from build123d import *

# Parameters (mm, degrees)
SKETCH1_R           = 10
BOSS_EXTRUDE1_DEPTH = 10


with BuildPart() as part:
    # Sketch1 → Boss-Extrude1 (new body)
    with BuildSketch(Plane.XY):
        with BuildLine():
            Line((-89.519341996, 20), (310.480658004, 20))
            ThreePointArc((310.480658004, 20), (330.480658004, 0), (310.480658004, -20))
            Line((310.480658004, -20), (-89.519341996, -20))
            ThreePointArc((-89.519341996, -20), (-109.519341996, 0), (-89.519341996, 20))
        make_face()
        with Locations((-89.519341996, 0)):
            Circle(SKETCH1_R, mode=Mode.SUBTRACT)
        with Locations((310.480658004, 0)):
            Circle(SKETCH1_R, mode=Mode.SUBTRACT)
        with BuildLine():
            Line((10.480658004, 10), (210.480658004, 10))
            ThreePointArc((210.480658004, 10), (220.480658004, 0), (210.480658004, -10))
            Line((210.480658004, -10), (10.480658004, -10))
            ThreePointArc((10.480658004, -10), (0.480658004, 0), (10.480658004, 10))
        make_face(mode=Mode.SUBTRACT)
    extrude(amount=BOSS_EXTRUDE1_DEPTH)


solid = part.part
Source: CAD feature listing. Evaluate the final solid. Frame: model axes, mm. A direction names the side the tool comes from. Round coordinates to 2 decimals unless told otherwise and drop trailing zeros. Loops run counter-clockwise (first coordinate to the right, second up) from the corner with the lowest first, then second, coordinate; pieces in that order, holes last. Notation, with made-up numbers: (-31.5, -7) -> (-4.5, -7) arc R36 ccw to (-4.5, 32) -> close; hole circle Ø10 at (4, 47). An arc over 180 degrees is marked (long way). Answer as a JSON object with one key per item and string values. Group by question number.
Q1. Ray query, line 1 (Y direction, x = 49, z = 0.5); line 2 (X direction, y = 3.5, z = 5.25); line 3 (X direction, y = -1.5, z = 6.5). Return the intervals inside material, ascending. Write a range as from..to.
Q2. Section query C-C (z = 8.5). Output: boundary loops of the cut face in (x, y), plus the area to 3 significant figures.
Q3. Access query for faces 1 (the flat face through (108, 20, 5)), 2 (the flat face through (109, 10, 5)). Directions: +Z, -Z, +X, -X, +Y, -Y. A direction counts if a zero-diameter tool reaches every point of the face in a straight line with its end or side. Return the directions, or none.
Q4. Section query B-B (y = 0). Output: boundary loops of the cut face in (x, z).
Q5. Section query A-A (x = 202). Output: boundary loops of the cut face in (y, z).
Q6. Mould query, pull axis X, two halves, no side actions, for faces 3 (the flat face through (112, -10, 5)), 4 (the flat face through (114, 14, 10)), 5 (the cylindrical face through (-109.515, -0.44, 4.93)). Classes: pulls with the +X half, pulls with the -X half, needs draft (parallel to the pull), parting line crosses it, or undercut.
Q7. Contact query for a flat-ended pin moving along its axis: P1, Ø1.5, axis at y = -2, z = 1.5, coming from the -X side. Output: stop coordinate, or through.
Completed:
{
 "1": {"line 1": "-20..-10, 10..20", "line 2": "-109.21..-98.89, -80.15..1.11, 219.85..301.11, 319.85..330.17", "line 3": "-109.46..-99.41, -79.63..0.59, 220.37..300.59, 320.37..330.42"},
 "2": {"outline": "(-89.52, -20) -> (310.48, -20) arc R20 ccw to (310.48, 20) -> (-89.52, 20) arc R20 ccw to start; hole circle Ø20 at (-89.52, 0); hole (10.48, -10) -> (210.48, -10) arc R10 ccw to (210.48, 10) -> (10.48, 10) arc R10 ccw to start; hole circle Ø20 at (310.48, 0)", "area": "12,300 mm²"},
 "3": {"face 1": "+Z, -Z, +X, -X, +Y", "face 2": "+Z, -Z"},
 "4": {"outline": "(-109.52, 0) -> (-99.52, 0) -> (-99.52, 10) -> (-109.52, 10) -> close; (-79.52, 0) -> (0.48, 0) -> (0.48, 10) -> (-79.52, 10) -> close; (220.48, 0) -> (300.48, 0) -> (300.48, 10) -> (220.48, 10) -> close; (320.48, 0) -> (330.48, 0) -> (330.48, 10) -> (320.48, 10) -> close"},
 "5": {"outline": "(-20, 0) -> (-10, 0) -> (-10, 10) -> (-20, 10) -> close; (10, 0) -> (20, 0) -> (20, 10) -> (10, 10) -> close"},
 "6": {"face 3": "undercut", "face 4": "needs draft", "face 5": "pulls with the -X half"},
 "7": {"P1": "x = -109.48"}
}
